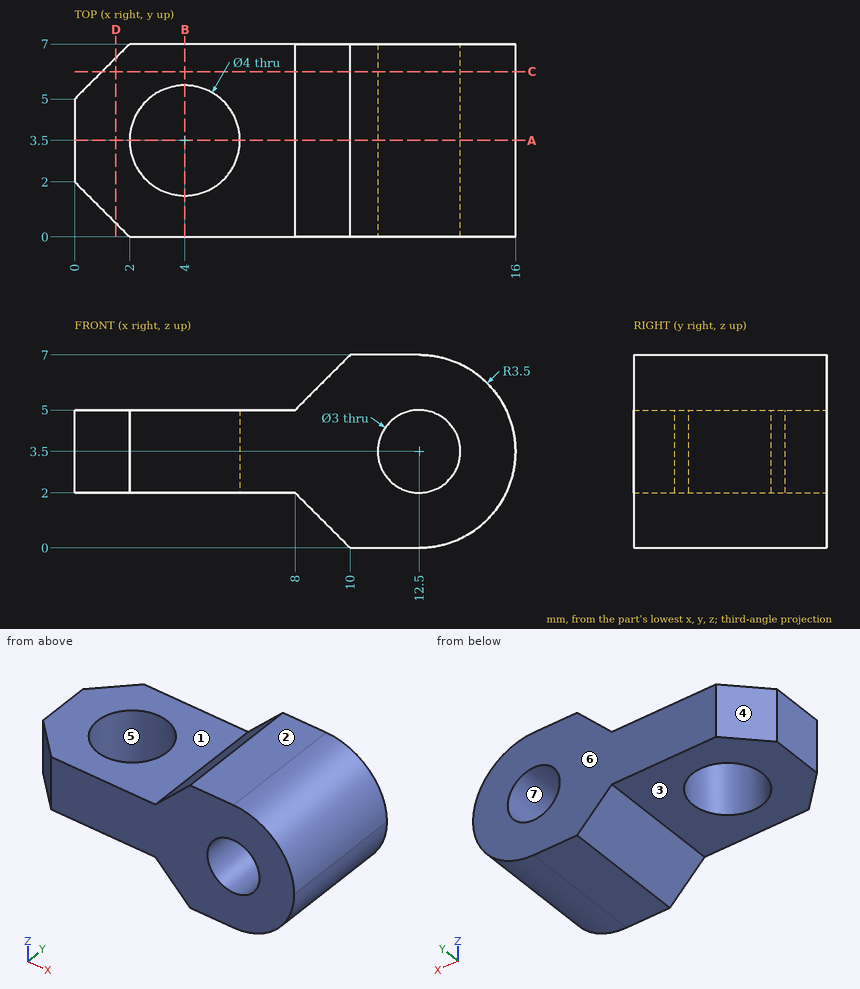
Here's the drawing with two shaded views (mm, measured from the low corner). I have some questions. A direction names the side the tool comes from. Round coordinates to 2 decimals unless told otherwise and drop trailing zeros. Order: outer loops, then holes, each group sorted by start corner. A loop starts at its lowest first (then second) coordinate and runs counter-clockwise, first axis right, second up. Notation, with made-up numbers: (65, 36.5) -> (86, 36.5) arc R25 cw to (86, 55.5) -> close; hole circle Ø1 at (-12, 29.25). An arc over 180 degrees is marked (long way). Use a Markdown table: item, result. Add a question column.
(1) Suppose I cut it at A-A, the plane y = 3.5. Please give me the cut outline in (x, z).
(2) Suppose I cut it at D-D, the plane x = 1.5. Please give me the cut outline in (y, z).
(3) Suppose I cut it at C-C, the plane y = 6. Please give me the cut outline in (x, z), and give its area (3 significant figures).
(4) For pin 1 Ø3 at (y, z) = (5, 1) entering from +X; pin 2 Ø2 at (x, y) = (4.5, 2) entering from -Z, each with a flat end and sliding along its axis, tell me the tip position at first contact or that it passes through.
(5) Suppose I cut it at B-B, the plane x = 4. Please give me the cut outline in (y, z), and give its area (3 significant figures).
(6) If we mould it in two halves opening along X, with no side actions, what happens to the marked faces 4, 5, 6 and 7? For each: released by +X, released by -X, zero draft, split by the parting line, or undercut.
(7) I need wall thicknesses on line 1 along Z through (x, y) = (12.5, 1.75); line 2 along X through (y, z) = (3, 2.5); line 3 along X through (y, z) = (3, 3). Which ranges of each line are inside material? Lowest first, please.
(8) For the marked faces 1, 2 and 3, which set-ups out of +Z, -Z, +X, -X, +Y, -Y let a thin tool reach every point of the face, with its end or its side?
Verdict:
| question | item | result |
|---|---|---|
| 1 | outline | (0, 2) -> (2, 2) -> (2, 5) -> (0, 5) -> close; (6, 2) -> (8, 2) -> (10, 0) -> (12.5, 0) arc R3.5 ccw to (16, 3.5) arc R3.5 ccw to (12.5, 7) -> (10, 7) -> (8, 5) -> (6, 5) -> close; hole circle Ø3 at (12.5, 3.5) |
| 2 | outline | (0.5, 2) -> (6.5, 2) -> (6.5, 5) -> (0.5, 5) -> close |
| 3 | outline | (1, 2) -> (8, 2) -> (10, 0) -> (12.5, 0) arc R3.5 ccw to (16, 3.5) arc R3.5 ccw to (12.5, 7) -> (10, 7) -> (8, 5) -> (1, 5) -> close; hole circle Ø3 at (12.5, 3.5) |
| 3 | area | 60.7 mm2 |
| 4 | pin 1 | x = 15.85 |
| 4 | pin 2 | z = 2 |
| 5 | outline | (0, 2) -> (1.5, 2) -> (1.5, 5) -> (0, 5) -> close; (5.5, 2) -> (7, 2) -> (7, 5) -> (5.5, 5) -> close |
| 5 | area | 9.00 mm2 |
| 6 | face 4 | released by -X |
| 6 | face 5 | undercut |
| 6 | face 6 | zero draft |
| 6 | face 7 | undercut |
| 7 | line 1 | 0 to 2, 5 to 7 |
| 7 | line 2 | 0 to 2.06, 5.94 to 11.38, 13.62 to 15.85 |
| 7 | line 3 | 0 to 2.06, 5.94 to 11.09, 13.91 to 15.96 |
| 8 | face 1 | +Z, -X, +Y, -Y |
| 8 | face 2 | +Z, +X, -X, +Y, -Y |
| 8 | face 3 | -Z, -X, +Y, -Y |
